```python
from build123d import *

# Parameters (mm, degrees)
SKETCH1_W           = 60
SKETCH1_H           = 60
BOSS_EXTRUDE1_DEPTH = 6
SKETCH2_W           = 10
SKETCH2_H           = 6
BOSS_EXTRUDE2_DEPTH = 14
BOSS_EXTRUDE3_DEPTH = 10
SKETCH4_R           = 3.625
CUT_EXTRUDE1_DEPTH  = 15
LPATTERN2_COUNT     = 3
LPATTERN2_PITCH     = 25
SKETCH5_R           = 1.625
CUT_EXTRUDE2_DEPTH  = 15
CIRPATTERN2_COUNT   = 6
FILLET1_R           = 20
SKETCH_3_W          = 65
SKETCH_3_H          = 40
SKETCH_3_R          = 3.625
EXTRUDE_1_DEPTH     = 6
SKETCH_6_W          = 15.5
SKETCH_6_H          = 6
CUT_EXTRUDE_2_DEPTH = 65
FILLET_2_R          = 2.5
SKETCH_7_W          = 2
SKETCH_7_H          = 4
CUT_EXTRUDE_3_DEPTH = 10


with BuildPart() as part:
    # Sketch1 → Boss-Extrude1 (new body)
    with BuildSketch(Plane.XY):
        Rectangle(SKETCH1_W, SKETCH1_H)
    extrude(amount=BOSS_EXTRUDE1_DEPTH)

    # Sketch2 → Boss-Extrude2 (add)
    with BuildSketch(Plane.XY.offset(6)):
        with Locations((25, -27)):
            Rectangle(SKETCH2_W, SKETCH2_H)
    boss_extrude2 = extrude(amount=BOSS_EXTRUDE2_DEPTH)

    # Sketch3 → Boss-Extrude3 (add)
    with BuildSketch(Plane(origin=(30, 0, 0), x_dir=(0, 0, -1), z_dir=(1, 0, 0))):
        Polygon((-6, -18), (-9, -24), (-6, -24), align=None)
        Polygon((0, -20), (2, -24), (0, -24), align=None)
    boss_extrude3 = extrude(amount=-BOSS_EXTRUDE3_DEPTH)

    # Sketch4 → Cut-Extrude1 (cut)
    with BuildSketch(Plane(origin=(0, -24, 0), x_dir=(1, 0, 0), z_dir=(0, 1, 0))):
        with Locations((25, -15)):
            Circle(SKETCH4_R)
    cut_extrude1 = extrude(amount=-CUT_EXTRUDE1_DEPTH, mode=Mode.SUBTRACT)

    # LPattern2: Boss-Extrude2, Boss-Extrude3, Cut-Extrude1 ×3
    with Locations(*[(-i * LPATTERN2_PITCH, 0, 0) for i in range(1, LPATTERN2_COUNT)]):
        add(boss_extrude2)
        add(boss_extrude3)
        add(cut_extrude1, mode=Mode.SUBTRACT)

    # Sketch5 → Cut-Extrude2 (cut)
    with BuildSketch(Plane(origin=(0, 0, 0), x_dir=(-1, 0, 0), z_dir=(0, 0, -1))):
        with Locations((3.406977246, 23.321928114)):
            Circle(SKETCH5_R)
        with Locations((-3.406977246, 23.321928114)):
            Circle(SKETCH5_R)
    cut_extrude2 = extrude(amount=-CUT_EXTRUDE2_DEPTH, mode=Mode.SUBTRACT)

    # CirPattern2: Cut-Extrude2 ×6 about axis
    cirpattern2_axis = Axis((0, 4, 0), (0, 0, 1))
    for i in range(1, CIRPATTERN2_COUNT):
        add(cut_extrude2.rotate(cirpattern2_axis, i * 360 / CIRPATTERN2_COUNT), mode=Mode.SUBTRACT)

    # Fillet1
    fillet1_edges = [part.edges().sort_by_distance(p)[0] for p in [
        (-30, 30, 3),
        (30, 30, 3),
    ]]
    fillet(fillet1_edges, radius=FILLET1_R)

    # 스케치3 → 보스-돌출1 (add)
    with BuildSketch(Plane.XZ.offset(30)):
        with Locations((0, 2.5)):
            Rectangle(SKETCH_3_W, SKETCH_3_H)
        with Locations((-25, 15)):
            Circle(SKETCH_3_R, mode=Mode.SUBTRACT)
        with Locations((0, 15)):
            Circle(SKETCH_3_R, mode=Mode.SUBTRACT)
        with Locations((25, 15)):
            Circle(SKETCH_3_R, mode=Mode.SUBTRACT)
        with Locations((-25, -10)):
            Circle(SKETCH_3_R, mode=Mode.SUBTRACT)
        with Locations((0, -10)):
            Circle(SKETCH_3_R, mode=Mode.SUBTRACT)
        with Locations((25, -10)):
            Circle(SKETCH_3_R, mode=Mode.SUBTRACT)
    extrude(amount=-EXTRUDE_1_DEPTH)

    # 스케치6 → 컷-돌출2 (cut)
    with BuildSketch(Plane(origin=(32.5, 0, 0), x_dir=(0, 0, -1), z_dir=(1, 0, 0))):
        with Locations((9.75, -27)):
            Rectangle(SKETCH_6_W, SKETCH_6_H)
    extrude(amount=-CUT_EXTRUDE_2_DEPTH, mode=Mode.SUBTRACT)

    # 필렛2
    fillet_2_edges = [part.edges().sort_by_distance(p)[0] for p in [
        (-32.5, -27, 22.5),
        (-32.5, -27, -2),
        (32.5, -27, 22.5),
        (32.5, -27, -2),
    ]]
    fillet(fillet_2_edges, radius=FILLET_2_R)

    # 스케치7 → 컷-돌출3 (cut)
    with BuildSketch(Plane(origin=(5, 0, 0), x_dir=(0, 0, -1), z_dir=(1, 0, 0))):
        with Locations((1, -22)):
            Rectangle(SKETCH_7_W, SKETCH_7_H)
    extrude(amount=-CUT_EXTRUDE_3_DEPTH, mode=Mode.SUBTRACT)


solid = part.part
```
The listing builds one solid part. Answer for the finished solid, in the listing's coordinates (mm). A direction names the side the tool comes from. Coordinates: 2 decimals unless noted, no trailing zeros. Write each loop counter-clockwise with the first axis right and the second up, starting at its lowest first coordinate (ties: lowest second). Pieces come first, ordered by that corner, then holes.
Q1. Which of the six approach directions +Z, -Z, +X, -X, +Y, -Y give full straight-line access (tool end or side, diameter ignored) to faces 4 (the flat face through (5, -22, 7)), 5 (the cylindrical face through (-24.297, 23.986, 3.042)), 6 (the flat face through (-20, -23, -1))?
Returned:
face 4: +Z, +Y
face 5: +Z, -Z, -X, +Y
face 6: -Z, +Y
Q2. The mould has two halves that part along X. Classify faces 1 (the cylindrical face through (31.748, -26.958, 21.787)), 2 (the flat face through (-24.9, -21, 7.5)), 3 (the cylindrical face through (13.74, 17.6, 2.96)): released by +X, released by -X, zero draft, split by the parting line, or undercut.
Returned:
face 1: released by +X
face 2: zero draft
face 3: undercut
Q3. Given P1, Ø3.5, axis at y = -21.5, z = 7.5, coming from the -X side; P2, Ø5, axis at x = -15.03, y = 16.61, coming from the +Z side; P3, Ø2.5, axis at y = -21.5, z = 7.5, coming from the +X side, each flat-ended and moving along its own axis, determine where each tip first touches the part or whether it passes through.
Returned:
P1: stops at x = -30
P2: stops at z = 6
P3: stops at x = 30
Q4. Section A-A, the plane x = 0 is taken. Write down the section's boundary in (y, z) (3 decimals), then the cut area to 4 significant figures.
Returned:
outline: (-30, -2) - (-24, -2) - (-24, 0) - (30, 0) - (30, 6) - (-18, 6) - (-24, 9) - (-24, 11.375) - (-30, 11.375) - close; (-30, 18.625) - (-24, 18.625) - (-24, 22.5) - (-30, 22.5) - close
area: 436.5 mm2
Q5. Section D-D, the plane y = -21 is taken. Write down the section's boundary in (x, z), then the cut area to 3 significant figures.
Returned:
outline: (-30, -0.5) - (-20, -0.5) - (-20, 0) - (20, 0) - (20, -0.5) - (30, -0.5) - (30, 7.5) - (20, 7.5) - (20, 6) - (5, 6) - (5, 7.5) - (-5, 7.5) - (-5, 6) - (-20, 6) - (-20, 7.5) - (-30, 7.5) - close
area: 415 mm2
Q6. Find the intervals of material crossed by line 1 along X through (y, z) = (-28.3, 15) (3 decimals); line 2 along Y through (x, z) = (-15.5, 2.5); line 3 along Z through (x, y) = (15, -18.5), in increasing order.
Returned:
line 1: x = -32.5 to -28.625, -21.375 to -3.625, 3.625 to 21.375, 28.625 to 32.5
line 2: y = -30 to -10.17, -7.06 to 15.06, 18.17 to 29.23
line 3: z = 0 to 6
Q7. Section B-B, the plane z = 15 is taken. Write down the section's boundary in (x, y) (3 decimals), then the cut area to 4 significant figures.
Returned:
outline: (-32.5, -30) - (-28.625, -30) - (-28.625, -24) - (-32.5, -24) - close; (-21.375, -30) - (-3.625, -30) - (-3.625, -24) - (-21.375, -24) - close; (3.625, -30) - (21.375, -30) - (21.375, -24) - (3.625, -24) - close; (28.625, -30) - (32.5, -30) - (32.5, -24) - (28.625, -24) - close
area: 259.5 mm2
Q8. Section C-C, the plane y = 17 is taken. Write down the section's boundary in (x, z) (3 decimals), then the cut area to 3 significant figures.
Returned:
outline: (-28.735, 0) - (-16.608, 0) - (-16.608, 6) - (-28.735, 6) - close; (-13.452, 0) - (13.452, 0) - (13.452, 6) - (-13.452, 6) - close; (16.608, 0) - (28.735, 0) - (28.735, 6) - (16.608, 6) - close
area: 307 mm2
